Geometry check sheet. Reference: the model listing, model coordinates, mm. A direction names the side the tool comes from. Round coordinates to 2 decimals unless told otherwise and drop trailing zeros. Write each loop counter-clockwise with the first axis right and the second up, starting at its lowest first coordinate (ties: lowest second). Pieces come first, ordered by that corner, then holes.
Item 1: Cross-section at A-A (z = 0). Enter the section's corners in (x, y), then the cut area to 3 significant figures.
Item 2: Cross-section at B-B (x = -9.5). Enter the section's corners in (y, z), then the cut area to 3 significant figures.
Item 3: Cross-section at D-D (x = 10.5). Enter the section's corners in (y, z), then the cut area to 3 significant figures.
Item 4: Depth check by flat-ended pin: P1, Ø1.8, axis at x = 2, y = -3, coming from the +Z side; P2, Ø6.5, axis at x = -11, z = 0, coming from the -Y side; P3, Ø0.5, axis at x = -12.5, z = -10, coming from the -Y side. Enter the tip coordinate at first touch or a pass-through.
Item 5: Access from +Z, -Z, +X, -X, +Y, -Y to the whole of each face (thin tool, end or side, straight path). Record for faces 1 (the face through (7.493, -6, -13)), 2 (the face through (0, 0, -1)), 3 (the face through (0, -3, -11.176)).
Item 6: Draft check along Z on faces 4 (the face through (0.1, -7.24, -13.01)), 5 (the face through (-8.94, 0.75, 0.46)), 6 (the face through (11, -2.032, -10)), 7 (the face through (0.21, -0.58, -9.04)). Enter one of: pulls with the +Z half, pulls with the -Z half, needs draft (parallel to the pull), parting line crosses it, or undercut.
Item 7: Cross-section at C-C (x = 2). Enter the section's corners in (y, z) (3 decimals).
Item 8: Scan lines: probe 1 along X at (y, z) = (1.15, 0); probe 2 along Y at (x, z) = (-4.5, -1.5); probe 3 along Z at (x, y) = (4, -2). Record each from-to range of solid material in increasing order.
from build123d import *

# Parameters (mm, degrees)
EXTRUDE1_DEPTH     = 14.986
SKETCH3_W          = 10.126198966
SKETCH3_H          = 9.525984496
CUT_EXTRUDE1_DEPTH = 24.44276897
SKETCH4_W          = 11.338244961
SKETCH4_H          = 6.180272868
SKETCH4_W_2        = 9.014834109
SKETCH4_H_2        = 6.970232558
CUT_EXTRUDE2_DEPTH = 24.44276897
CHAMFER1_SIZE      = 1.524
SKETCH5_R          = 2.1082
CUT_EXTRUDE3_DEPTH = 24.44276897


with BuildPart() as part:
    # Sketch2 → Extrude1 (new, symmetric)
    with BuildSketch(Plane(origin=(0, 0, 0), x_dir=(0, 0, -1), z_dir=(1, 0, 0))):
        with BuildLine():
            Line((-5.334, 0), (7.62, 0))
            ThreePointArc((7.62, 0), (9.056840979, -0.595159021), (9.652, -2.032))
            Line((9.652, -2.032), (9.652, -3.81))
            ThreePointArc((9.652, -3.81), (13.081, -7.239), (16.51, -3.81))
            Line((16.51, -3.81), (16.51, -1.524))
            Line((16.51, -1.524), (14.986, -1.524))
            Line((14.986, -1.524), (14.986, -3.81))
            ThreePointArc((14.986, -3.81), (13.081, -5.715), (11.176, -3.81))
            Line((11.176, -3.81), (11.176, -2.032))
            ThreePointArc((11.176, -2.032), (10.134471714, 0.482471714), (7.62, 1.524))
            Line((7.62, 1.524), (-5.334, 1.524))
            Line((-5.334, 1.524), (-5.334, 0))
        make_face()
    extrude(amount=EXTRUDE1_DEPTH, both=True)

    # Sketch3 → Cut-Extrude1 (cut, through all)
    with BuildSketch(Plane.XY):
        with Locations((-12.556099483, -6.794992248)):
            Rectangle(SKETCH3_W, SKETCH3_H)
        with Locations((12.556099483, -6.794992248)):
            Rectangle(SKETCH3_W, SKETCH3_H)
    extrude(amount=-CUT_EXTRUDE1_DEPTH, mode=Mode.SUBTRACT)

    # Sketch4 → Cut-Extrude2 (cut, through all)
    with BuildSketch(Plane(origin=(0, 0, 0), x_dir=(1, 0, 0), z_dir=(0, 1, 0))):
        with Locations((-13.16212248, 16.740372093)):
            Rectangle(SKETCH4_W, SKETCH4_H)
        with Locations((12.000417055, 16.577733333)):
            Rectangle(SKETCH4_W_2, SKETCH4_H_2)
    extrude(amount=-CUT_EXTRUDE2_DEPTH, mode=Mode.SUBTRACT)

    # Chamfer1
    chamfer1_edges = [part.edges().sort_by_distance(p)[0] for p in [
        (7.493, -1.524, -15.748),
        (-7.493, -1.524, -15.748),
    ]]
    chamfer(chamfer1_edges, length=CHAMFER1_SIZE)

    # Sketch5 → Cut-Extrude3 (cut, through all)
    with BuildSketch(Plane(origin=(0, 0, 0), x_dir=(1, 0, 0), z_dir=(0, 1, 0))):
        with Locations(Location((10.9982, 0, 0), (0, 0, 270))):
            Circle(SKETCH5_R)
        with Locations(Location((-10.9982, 0, 0), (0, 0, 90))):
            Circle(SKETCH5_R)
    extrude(amount=CUT_EXTRUDE3_DEPTH, mode=Mode.SUBTRACT)


solid = part.part
Resolved:
1. outline: (-14.99, 0) - (-13.11, 0) - (-13.11, 1.52) - (-14.99, 1.52) - close; (-8.89, 0) - (8.89, 0) - (8.89, 1.52) - (-8.89, 1.52) - close; (13.11, 0) - (14.99, 0) - (14.99, 1.52) - (13.11, 1.52) - close
1. area: 32.8 mm2
2. outline: (-2.03, -11.18) arc R3.56 ccw to (1.52, -7.62) - (1.52, -1.48) - (0, -1.48) - (0, -7.62) arc R2.03 cw to (-2.03, -9.65) - close; (0, 1.48) - (1.52, 1.48) - (1.52, 5.33) - (0, 5.33) - close
2. area: 21.9 mm2
3. outline: (-2.03, -11.18) arc R3.56 ccw to (1.52, -7.62) - (1.52, -2.05) - (0, -2.05) - (0, -7.62) arc R2.03 cw to (-2.03, -9.65) - close; (0, 2.05) - (1.52, 2.05) - (1.52, 5.33) - (0, 5.33) - close
3. area: 20.2 mm2
4. P1: stops at z = -9.65
4. P2: stops at y = 0
4. P3: stops at y = -2.03
5. face 1: +Z, -Z, +X, -Y
5. face 2: +Z, +X, -X, -Y
5. face 3: +X, -X, +Y
6. face 4: parting line crosses it
6. face 5: undercut
6. face 6: needs draft
6. face 7: pulls with the +Z half
7. outline: (-3.81, -16.51) - (-1.524, -16.51) - (-1.524, -14.986) - (-3.81, -14.986) arc R1.905 cw to (-3.81, -11.176) - (-2.032, -11.176) arc R3.556 ccw to (1.524, -7.62) - (1.524, 5.334) - (0, 5.334) - (0, -7.62) arc R2.032 cw to (-2.032, -9.652) - (-3.81, -9.652) arc R3.429 ccw to start
8. probe 1: x = -14.99 to -13.11, -8.89 to 8.89, 13.11 to 14.99
8. probe 2: y = 0 to 1.52
8. probe 3: z = -16.51 to -14.99, -11.18 to -9.65
